Design review of the part built by this model. Coordinates are the model's own, in mm. A direction names the side the tool comes from. Coordinates: 2 decimals unless noted, no trailing zeros. Order: outer loops, then holes, each group sorted by start corner. A loop starts at its lowest first (then second) coordinate and runs counter-clockwise, first axis right, second up. Notation, with made-up numbers: (14.25, 7) -> (43.25, 7) arc R15 ccw to (43.25, 22) -> close; hole circle Ø3 at (85.25, 28.5). An arc over 180 degrees is marked (long way). Write item = value, one per line.
```python
from build123d import *

# Parameters (mm, degrees)
SKETCH1_W           = 46.4
SKETCH1_H           = 5.9
SKETCH1_W_2         = 42
SKETCH1_H_2         = 3.5
BOSS_EXTRUDE1_DEPTH = 32.25
FILLET2_R           = 3
SKETCH2_W           = 54
SKETCH2_H           = 13.5
SKETCH2_W_2         = 42
SKETCH2_H_2         = 3.5
BOSS_EXTRUDE2_DEPTH = 5.8
SKETCH3_W           = 54
SKETCH3_H           = 13.5
SKETCH3_W_2         = 42
SKETCH3_H_2         = 3.5
BOSS_EXTRUDE3_DEPTH = 5.8
SKETCH4_R           = 1.6
CUT_EXTRUDE1_DEPTH  = 65.421211569
SKETCH15_W          = 42
SKETCH15_H          = 3.5
SKETCH15_W_2        = 5.8
SKETCH15_H_2        = 2
CUT_EXTRUDE5_DEPTH  = 68.356903878
FILLET3_R           = 2
SKETCH16_W          = 42
SKETCH16_H          = 1.2
BOSS_EXTRUDE4_DEPTH = 26
SKETCH16_3_W        = 5.8
SKETCH16_3_H        = 2
BOSS_EXTRUDE5_DEPTH = 30
SKETCH17_W          = 29
SKETCH17_H          = 32
CUT_EXTRUDE6_DEPTH  = 10
CUT_EXTRUDE7_DEPTH  = 30
SKETCH19_W          = 3.6
SKETCH19_H          = 32
BOSS_EXTRUDE6_DEPTH = 3.8
SKETCH20_R          = 1.5
CUT_EXTRUDE8_DEPTH  = 88.534179039


with BuildPart() as part:
    # Sketch1 → Boss-Extrude1 (new body)
    with BuildSketch(Plane(origin=(0, 0, 0), x_dir=(0, 0, -1), z_dir=(1, 0, 0))):
        with Locations((23.2, 2.95)):
            Rectangle(SKETCH1_W, SKETCH1_H)
        with Locations((23.2, 2.95)):
            Rectangle(SKETCH1_W_2, SKETCH1_H_2, mode=Mode.SUBTRACT)
    extrude(amount=BOSS_EXTRUDE1_DEPTH)

    # Fillet2
    # the kernel refuses this fillet: 3 mm, written as the material it takes off along each edge
    with BuildSketch(Plane(origin=(-7.5, 0, -46.4), x_dir=(0, 0, 1), z_dir=(1, 0, 0)), Plane(origin=(-7.5, 5.9, 0), x_dir=(0, 0, -1), z_dir=(1, 0, 0)), Plane(origin=(-7.5, 5.9, -46.4), x_dir=(0, -1, 0), z_dir=(1, 0, 0))) as fillet2_piece_1:
        with BuildLine():
            CenterArc((FILLET2_R, -FILLET2_R), FILLET2_R, 90, 90)
            Line((0, -FILLET2_R), (0, 0))
            Line((0, 0), (FILLET2_R, 0))
        make_face()
    extrude(amount=47.25, mode=Mode.SUBTRACT)
    with BuildSketch(Plane(origin=(-7.5, 0, 0), x_dir=(0, 0, -1), z_dir=(1, 0, 0))) as fillet2_piece_2:
        with BuildLine():
            CenterArc((FILLET2_R, FILLET2_R), FILLET2_R, 180, 90)
            Line((0, FILLET2_R), (0, 0))
            Line((0, 0), (FILLET2_R, 0))
        make_face()
    extrude(amount=47.25, mode=Mode.SUBTRACT)

    # Sketch2 → Boss-Extrude2 (add)
    with BuildSketch(Plane(origin=(32.25, 0, 0), x_dir=(0, 0, -1), z_dir=(1, 0, 0))):
        with Locations((23.2, 2.95)):
            Rectangle(SKETCH2_W, SKETCH2_H)
        with Locations((23.2, 2.95)):
            Rectangle(SKETCH2_W_2, SKETCH2_H_2, mode=Mode.SUBTRACT)
    extrude(amount=BOSS_EXTRUDE2_DEPTH)

    # Sketch3 → Boss-Extrude3 (add)
    with BuildSketch(Plane.ZY):
        with Locations((-23.2, 2.95)):
            Rectangle(SKETCH3_W, SKETCH3_H)
        with Locations((-23.2, 2.95)):
            Rectangle(SKETCH3_W_2, SKETCH3_H_2, mode=Mode.SUBTRACT)
    extrude(amount=BOSS_EXTRUDE3_DEPTH)

    # Sketch4 → Cut-Extrude1 (cut, through all)
    with BuildSketch(Plane(origin=(0, 9.7, 0), x_dir=(1, 0, 0), z_dir=(0, 1, 0))):
        with Locations(Location((-2.9, 47.3, 0), (0, 0, 270))):
            Circle(SKETCH4_R)
        with Locations(Location((35.15, 47.3, 0), (0, 0, 270))):
            Circle(SKETCH4_R)
        with Locations(Location((-2.9, -0.9, 0), (0, 0, 270))):
            Circle(SKETCH4_R)
        with Locations(Location((35.15, -0.9, 0), (0, 0, 270))):
            Circle(SKETCH4_R)
    extrude(amount=-CUT_EXTRUDE1_DEPTH, mode=Mode.SUBTRACT)

    # Sketch15 → Cut-Extrude5 (cut, through all)
    with BuildSketch(Plane.ZY.offset(5.8)):
        with Locations((-23.2, 2.95)):
            Rectangle(SKETCH15_W, SKETCH15_H)
        with Locations((-47.3, -2.8)):
            Rectangle(SKETCH15_W_2, SKETCH15_H_2)
        with Locations((0.9, -2.8)):
            Rectangle(SKETCH15_W_2, SKETCH15_H_2)
    extrude(amount=-CUT_EXTRUDE5_DEPTH, mode=Mode.SUBTRACT)

    # Fillet3
    fillet3_edges = [part.edges().sort_by_distance(p)[0] for p in [
        (-5.8, -3.8, -23.2),
    ]]
    fillet(fillet3_edges, radius=FILLET3_R)

    # Sketch16 → Boss-Extrude4 (add)
    with BuildSketch(Plane(origin=(38.05, 0, 0), x_dir=(0, 0, -1), z_dir=(1, 0, 0))):
        with Locations((23.2, 0.6)):
            Rectangle(SKETCH16_W, SKETCH16_H)
    extrude(amount=BOSS_EXTRUDE4_DEPTH)

    # Sketch16<3> → Boss-Extrude5 (add)
    with BuildSketch(Plane(origin=(38.05, 0, 0), x_dir=(0, 0, -1), z_dir=(1, 0, 0))):
        Polygon((2, -1.8), (2, -3.8), (44.4, -3.8), (44.4, -1.8), (50.2, -1.8), (50.2, 0), (44.2, 0), (2.2, 0), (-3.8, 0), (-3.8, -1.8), align=None)
        with Locations((-0.9, -2.8)):
            Rectangle(SKETCH16_3_W, SKETCH16_3_H)
        with Locations((47.3, -2.8)):
            Rectangle(SKETCH16_3_W, SKETCH16_3_H)
    extrude(amount=BOSS_EXTRUDE5_DEPTH)

    # Sketch17 → Cut-Extrude6 (cut)
    with BuildSketch(Plane(origin=(0, 1.2, 0), x_dir=(1, 0, 0), z_dir=(0, 1, 0))):
        with Locations((53.55, 23.2)):
            Rectangle(SKETCH17_W, SKETCH17_H)
    extrude(amount=-CUT_EXTRUDE6_DEPTH, mode=Mode.SUBTRACT)

    # Sketch18 → Cut-Extrude7 (cut)
    with BuildSketch(Plane.XZ.offset(3.8)):
        with BuildLine():
            ThreePointArc((39.184435563, 3.8), (39.00939278, 3.313556237), (38.95, 2.8))
            ThreePointArc((38.95, 2.8), (41.2, 0.55), (43.45, 2.8))
            ThreePointArc((43.45, 2.8), (43.39060722, 3.313556237), (43.215564437, 3.8))
            Line((43.215564437, 3.8), (39.184435563, 3.8))
        make_face()
        with BuildLine():
            ThreePointArc((43.215564437, 3.8), (41.2, 5.05), (39.184435563, 3.8))
            Line((39.184435563, 3.8), (43.215564437, 3.8))
        make_face()
        with BuildLine():
            Line((38.95, 3.8), (38.95, 2.8))
            ThreePointArc((38.95, 2.8), (39.00939278, 3.313556237), (39.184435563, 3.8))
            Line((39.184435563, 3.8), (38.95, 3.8))
        make_face()
        with BuildLine():
            ThreePointArc((43.215564437, 3.8), (43.39060722, 3.313556237), (43.45, 2.8))
            Line((43.45, 2.8), (43.45, 3.8))
            Line((43.45, 3.8), (43.215564437, 3.8))
        make_face()
        with BuildLine():
            ThreePointArc((43.45, -49.2), (41.2, -46.95), (38.95, -49.2))
            ThreePointArc((38.95, -49.2), (39.00939278, -49.713556237), (39.184435563, -50.2))
            Line((39.184435563, -50.2), (43.215564437, -50.2))
            ThreePointArc((43.215564437, -50.2), (43.39060722, -49.713556237), (43.45, -49.2))
        make_face()
        with BuildLine():
            Line((43.215564437, -50.2), (39.184435563, -50.2))
            ThreePointArc((39.184435563, -50.2), (41.2, -51.45), (43.215564437, -50.2))
        make_face()
        with BuildLine():
            ThreePointArc((39.184435563, -50.2), (39.00939278, -49.713556237), (38.95, -49.2))
            Line((38.95, -49.2), (38.95, -50.2))
            Line((38.95, -50.2), (39.184435563, -50.2))
        make_face()
        with BuildLine():
            Line((43.45, -50.2), (43.45, -49.2))
            ThreePointArc((43.45, -49.2), (43.39060722, -49.713556237), (43.215564437, -50.2))
            Line((43.215564437, -50.2), (43.45, -50.2))
        make_face()
    extrude(amount=-CUT_EXTRUDE7_DEPTH, mode=Mode.SUBTRACT)

    # Sketch19 → Boss-Extrude6 (add)
    with BuildSketch(Plane.XZ.offset(3.8)):
        with Locations((66.25, -23.2)):
            Rectangle(SKETCH19_W, SKETCH19_H)
        Polygon((71.05, 3.8), (68.05, 3.8), (68.05, -7.2), (68.05, -39.2), (68.05, -50.2), (71.05, -50.2), align=None)
    extrude(amount=-BOSS_EXTRUDE6_DEPTH)

    # Sketch20 → Cut-Extrude8 (cut, through all)
    with BuildSketch(Plane(origin=(0, 0, 0), x_dir=(1, 0, 0), z_dir=(0, 1, 0))):
        with Locations(Location((67.55, -0.3, 0), (0, 0, 270))):
            Circle(SKETCH20_R)
        with Locations(Location((67.55, 46.7, 0), (0, 0, 270))):
            Circle(SKETCH20_R)
    extrude(amount=-CUT_EXTRUDE8_DEPTH, mode=Mode.SUBTRACT)


solid = part.part
```
(1) For L1, parallel to Z at x = 67.55, y = -1.1; L2, parallel to X at y = 1.75, z = -47.3; L3, parallel to X at y = 8.5, z = -41.5, list the stretches that pass through material, from the lowest coordinate up.
Report:
L1 = -50.2 to -48.2, -45.2 to -1.2, 1.8 to 3.8
L2 = -5.8 to -4.5, -1.3 to 0, 32.25 to 33.55, 36.75 to 38.05
L3 = -5.8 to 0, 32.25 to 38.05
(2) We need section B-B (x = 67.55). Write out the cut boundary in (y, z), and give its area (3 significant figures).
Report:
outline = (-3.8, -50.2) -> (0, -50.2) -> (0, -48.2) -> (-3.8, -48.2) -> close; (-3.8, -45.2) -> (0, -45.2) -> (0, -1.2) -> (-3.8, -1.2) -> close; (-3.8, 1.8) -> (0, 1.8) -> (0, 3.8) -> (-3.8, 3.8) -> close
area = 182 mm²
(3) We need section D-D (x = 57). Write out the cut boundary in (y, z), and give its area (3 significant figures).
Report:
outline = (-3.8, -50.2) -> (0, -50.2) -> (0, -44.2) -> (1.2, -44.2) -> (1.2, -39.2) -> (-3.8, -39.2) -> close; (-3.8, -7.2) -> (1.2, -7.2) -> (1.2, -2.2) -> (0, -2.2) -> (0, 3.8) -> (-3.8, 3.8) -> close
area = 95.6 mm²
(4) We need section A-A (x = -2.9). Write out the cut boundary in (y, z), and give its area (3 significant figures).
Report:
outline = (-3.8, -44.4) -> (-1.8, -44.4) -> (-1.8, -45.7) -> (9.7, -45.7) -> (9.7, -0.7) -> (-1.8, -0.7) -> (-1.8, -2) -> (-3.8, -2) -> close; (-1.8, -50.2) -> (9.7, -50.2) -> (9.7, -48.9) -> (-1.8, -48.9) -> close; (-1.8, 2.5) -> (9.7, 2.5) -> (9.7, 3.8) -> (-1.8, 3.8) -> close; hole (1.2, -44.2) -> (4.7, -44.2) -> (4.7, -2.2) -> (1.2, -2.2) -> close
area = 485 mm²
(5) For faces 1 (the cylindrical face through (15.9, 5.06, -0.92)), 2 (the flat face through (35, -3, -2)), 3 (the flat face through (52, -1, -39.2)), 4 (the flat face through (21, 1.2, -23)), list the 3-axis set-ups (+Z, -Z, +X, -X, +Y, -Y) from which the entire face can be reached by the end or side of a thin tool; tool diameter is ignored.
Report:
face_1 = +Z, +Y
face_2 = +Z, -X, -Y
face_3 = +Y, -Y
face_4 = +X, -X
(6) Insertion check: pin 1 (1.5 mm diameter, centred on y = 8, z = -27.5, fed in from +X); pin 2 (6.5 mm diameter, centred on x = -2, z = -48, fed in from -Y); pin 3 (0.6 mm diameter, centred on y = 0.5, z = -4, fed in from +X); pin 4 (2.5 mm diameter, centred on x = 67.55, z = -46.7, fed in from -Y). Each pin has a flat end and moves straight along its axis. Give the tip position at first contact, or say it passes through.
Report:
pin_1 = 38.05
pin_2 = -1.8
pin_3 = 64.05
pin_4 = through
(7) We need section C-C (z = -32). Write out the cut boundary in (x, y).
Report:
outline = (-5.8, -1.8) arc R2 ccw to (-3.8, -3.8) -> (0, -3.8) -> (0, 0) -> (32.25, 0) -> (32.25, -3.8) -> (39.05, -3.8) -> (39.05, 1.2) -> (-5.8, 1.2) -> close; (-5.8, 4.7) -> (38.05, 4.7) -> (38.05, 9.7) -> (32.25, 9.7) -> (32.25, 5.9) -> (0, 5.9) -> (0, 9.7) -> (-5.8, 9.7) -> close; (64.45, -3.8) -> (71.05, -3.8) -> (71.05, 0) -> (64.45, 0) -> close
(8) The part is to be moulded in two halves that separate along Y. For faces 5 (the flat face through (-3, 9.7, -24)), 6 (the cylindrical face through (66.22, -1.87, -46.01)), 7 (the flat face through (16, 3, -44.2)), say which applies: released by +Y, released by -Y, zero draft, split by the parting line, or undercut.
Report:
face_5 = released by +Y
face_6 = zero draft
face_7 = undercut
